from build123d import *

# Parameters (mm, degrees)
F0_W     = 18.95
F0_H     = 18.95
F1_DEPTH = 4
F2_R     = 2
F3_SIZE  = 0.75


with BuildPart() as f1:
    # F0 (on Top) → F1 (new body)
    with BuildSketch(Plane.XY):
        Rectangle(F0_W, F0_H)
        Polygon((-6.47354, 0), (-3.23677, 5.60625), (3.23677, 5.60625), (6.47354, 0), (3.23677, -5.60625), (-3.23677, -5.60625), align=None, mode=Mode.SUBTRACT)
    extrude(amount=F1_DEPTH)

    # F2
    f2_edges = [f1.edges().sort_by_distance(p)[0] for p in [
        (9.475, -9.475, 2),
        (9.475, 9.475, 2),
        (-9.475, -9.475, 2),
        (-9.475, 9.475, 2),
    ]]
    fillet(f2_edges, radius=F2_R)

    # F3
    f3_edges = [f1.edges().sort_by_distance(p)[0] for p in [
        (9.475, 0, 4),
        (8.889214, -8.889214, 4),
        (8.889214, 8.889214, 4),
        (0, -9.475, 4),
        (0, 9.475, 4),
        (-8.889214, -8.889214, 4),
        (-8.889214, 8.889214, 4),
        (-9.475, 0, 4),
        (-4.855155, 2.803125, 4),
        (0, 5.60625, 4),
        (4.855155, 2.803125, 4),
        (4.855155, -2.803125, 4),
        (0, -5.60625, 4),
        (-4.855155, -2.803125, 4),
        (9.475, 0, 0),
        (8.889214, -8.889214, 0),
        (8.889214, 8.889214, 0),
        (0, -9.475, 0),
        (0, 9.475, 0),
        (-8.889214, -8.889214, 0),
        (-8.889214, 8.889214, 0),
        (-9.475, 0, 0),
        (-4.855155, 2.803125, 0),
        (0, 5.60625, 0),
        (4.855155, 2.803125, 0),
        (4.855155, -2.803125, 0),
        (0, -5.60625, 0),
        (-4.855155, -2.803125, 0),
    ]]
    chamfer(f3_edges, length=F3_SIZE)


solid = f1.part
Geometry check sheet. Reference: the model listing, model coordinates, mm. A direction names the side the tool comes from. Give positions to 0.01 mm unless a question says otherwise; leave off trailing zeros. Order: outer loops, then holes, each group sorted by start corner. A loop starts at its lowest first (then second) coordinate and runs counter-clockwise, first axis right, second up.
1. Scan lines: line 1 (Y direction, x = 0.5, z = 1.15) (3 decimals); line 2 (X direction, y = -4.75, z = 2.55) (3 decimals); line 3 (X direction, y = 4, z = 3.6) (3 decimals). Record each from-to range of solid material in increasing order.
Completed:
line 1: y = -9.475 to -5.606, 5.606 to 9.475
line 2: x = -9.475 to -3.731, 3.731 to 9.475
line 3: x = -9.125 to -4.568, 4.568 to 9.125
2. Sectioned sample at B-B (x = -0.25). Record the boundary of the cut face in (y, z) (3 decimals).
Completed:
outline: (-9.475, 0.75) - (-8.725, 0) - (-6.356, 0) - (-5.606, 0.75) - (-5.606, 3.25) - (-6.356, 4) - (-8.725, 4) - (-9.475, 3.25) - close; (5.606, 0.75) - (6.356, 0) - (8.725, 0) - (9.475, 0.75) - (9.475, 3.25) - (8.725, 4) - (6.356, 4) - (5.606, 3.25) - close
3. Draft check along Y on faces 1 (the face through (-8.56, 8.58, 3.7)), 2 (the face through (8.56, -8.58, 0.3)), 3 (the face through (5.15, 3.03, 0.38)). Enter one of: pulls with the +Y half, pulls with the -Y half, needs draft (parallel to the pull), parting line crosses it, or undercut.
Completed:
face 1: pulls with the +Y half
face 2: pulls with the -Y half
face 3: undercut
4. Sectioned sample at A-A (z = 1.7). Record the boundary of the cut face in (x, y) (3 decimals), then the cut area to 3 significant figures.
Completed:
outline: (-9.475, -7.475) arc R2 ccw to (-7.475, -9.475) - (7.475, -9.475) arc R2 ccw to (9.475, -7.475) - (9.475, 7.475) arc R2 ccw to (7.475, 9.475) - (-7.475, 9.475) arc R2 ccw to (-9.475, 7.475) - close; hole (-6.474, 0) - (-3.237, -5.606) - (3.237, -5.606) - (6.474, 0) - (3.237, 5.606) - (-3.237, 5.606) - close
area: 247 mm2
5. Sectioned sample at C-C (y = -1.5). Record the boundary of the cut face in (x, z) (3 decimals).
Completed:
outline: (-9.475, 0.75) - (-8.725, 0) - (-6.474, 0) - (-5.608, 0.75) - (-5.608, 3.25) - (-6.474, 4) - (-8.725, 4) - (-9.475, 3.25) - close; (5.608, 0.75) - (6.474, 0) - (8.725, 0) - (9.475, 0.75) - (9.475, 3.25) - (8.725, 4) - (6.474, 4) - (5.608, 3.25) - close
6. Access from +Z, -Z, +X, -X, +Y, -Y to the whole of each face (thin tool, end or side, straight path). Record for faces 4 (the face through (0, 5.606, 2)), 5 (the face through (-6, 4, 0)), 6 (the face through (5.201, -2.944, 3.62)).
Completed:
face 4: +Z, -Z
face 5: -Z, +X, -X, +Y, -Y
face 6: +Z
7. Sectioned sample at D-D (z = 0.5). Record the boundary of the cut face in (x, y) (3 decimals).
Completed:
outline: (-9.225, -7.475) arc R1.75 ccw to (-7.475, -9.225) - (7.475, -9.225) arc R1.75 ccw to (9.225, -7.475) - (9.225, 7.475) arc R1.75 ccw to (7.475, 9.225) - (-7.475, 9.225) arc R1.75 ccw to (-9.225, 7.475) - close; hole (-6.762, 0) - (-3.381, -5.856) - (3.381, -5.856) - (6.762, 0) - (3.381, 5.856) - (-3.381, 5.856) - close
